Check sheet for the modelled part. Datum: model origin and axes. Units: mm. Give positions to 0.01 mm unless a question says otherwise; leave off trailing zeros. Write each loop counter-clockwise with the first axis right and the second up, starting at its lowest first coordinate (ties: lowest second). Pieces come first, ordered by that corner, then holes. Notation, with made-up numbers: (42, 89) -> (99, 89) arc R7 ccw to (99, 98) -> close; hole circle Ø3 at (75, 3.5). An arc over 180 degrees is marked (long way). Return JSON: item names as keys, results as strings.
from build123d import *

# Parameters (mm, degrees)
SKETCH1_W             = 225.5266
SKETCH1_H             = 171.6532
BOSS_EXTRUDE1_DEPTH   = 3.175
SKETCH2_W             = 19.05
SKETCH2_H             = 19.05
SKETCH2_W_2           = 28.702
CORNERCUT_DEPTH       = 4.175
SKETCH3_R             = 2.4257
MOUNTHOLES_DEPTH      = 4.175
F_8_CLEARANCE_HOLE1_D = 4.4958


with BuildPart() as part:
    # Sketch1 → Boss-Extrude1 (new body)
    with BuildSketch(Plane(origin=(0, 0, 0), x_dir=(1, 0, 0), z_dir=(0, 1, 0))):
        Rectangle(SKETCH1_W, SKETCH1_H)
    extrude(amount=BOSS_EXTRUDE1_DEPTH)

    # Sketch2 → CornerCut (cut, through all)
    with BuildSketch(Plane(origin=(0, 3.175, 0), x_dir=(1, 0, 0), z_dir=(0, 1, 0))):
        with Locations((-103.2383, 76.3016)):
            Rectangle(SKETCH2_W, SKETCH2_H)
        with Locations((98.4123, -76.3016)):
            Rectangle(SKETCH2_W_2, SKETCH2_H)
        with Locations((-103.2383, -76.3016)):
            Rectangle(SKETCH2_W, SKETCH2_H)
    extrude(amount=-CORNERCUT_DEPTH, mode=Mode.SUBTRACT)

    # Sketch3 → MountHoles (cut, through all)
    with BuildSketch(Plane(origin=(0, 3.175, 0), x_dir=(1, 0, 0), z_dir=(0, 1, 0))):
        with Locations((-103.2383, 57.6834)):
            Circle(SKETCH3_R)
        with Locations((-103.2383, -57.6834)):
            Circle(SKETCH3_R)
        with Locations((93.5863, -57.6834)):
            Circle(SKETCH3_R)
        with Locations((103.6701, 57.6834)):
            Circle(SKETCH3_R)
    extrude(amount=-MOUNTHOLES_DEPTH, mode=Mode.SUBTRACT)

    # #8 Clearance Hole1 (through all)
    with Locations(Plane(origin=(0, 3.175, 0), x_dir=(1, 0, 0), z_dir=(0, 1, 0))):
        with Locations((-44.629848387, -79.4766), (-24.2443, 17.982191502), (-71.4883, 17.982191502)):
            Hole(F_8_CLEARANCE_HOLE1_D / 2)


solid = part.part
(1) Cross-section at B-B on z = -70.5. Enter the section's corners in (x, y) (3 decimals), then the cut area to 3 significant figures.
Reply:
{"outline": "(-93.713, 0) -> (112.763, 0) -> (112.763, 3.175) -> (-93.713, 3.175) -> close", "area": "656 mm^2"}
(2) Thickness scan on L1, parallel to Z at x = -24.5, y = 3; L2, parallel to X at y = 1.8, z = -20 (3 decimals); L3, parallel to X at y = 1.45, z = -56. Record the ranges inside material, lowest first.
Reply:
{"L1": "-85.83 to -20.22, -15.75 to 85.83", "L2": "-112.763 to -72.479, -70.498 to -25.235, -23.254 to 112.763", "L3": "-112.76 to -104.98, -101.49 to 101.92, 105.42 to 112.76"}
(3) Depth check by flat-ended pin: pin 1 Ø3.5 at (x, z) = (-71.49, -17.98) entering from +Y; pin 2 Ø1 at (y, z) = (2, -80.5) entering from -X; pin 3 Ø5 at (x, z) = (-44.63, 79.48) entering from +Y (3 decimals); pin 4 Ø1.6 at (x, y) = (-101, 2) entering from -Z. Enter the tip coordinate at first touch or a pass-through.
Reply:
{"pin 1": "through", "pin 2": "x = -93.71", "pin 3": "y = 3.175", "pin 4": "z = -66.78"}
(4) Release check for a two-part mould opening along Z. For faces 1 (the cylindrical face through (104.97, 1.61, -59.73)), 2 (the flat face through (-2, 0, -1)), 3 (the cylindrical face through (-69.243, 1.565, -18.081)) record: pulls with the +Z half, pulls with the -Z half, needs draft (parallel to the pull), parting line crosses it, or undercut.
Reply:
{"face 1": "undercut", "face 2": "needs draft", "face 3": "undercut"}
(5) Cross-section at A-A on y = 1.2. Enter the section's corners in (x, z).
Reply:
{"outline": "(-112.76, -66.78) -> (-93.71, -66.78) -> (-93.71, -85.83) -> (112.76, -85.83) -> (112.76, 66.78) -> (84.06, 66.78) -> (84.06, 85.83) -> (-93.71, 85.83) -> (-93.71, 66.78) -> (-112.76, 66.78) -> close; hole circle Ø4.85 at (-103.24, -57.68); hole circle Ø4.85 at (-103.24, 57.68); hole circle Ø4.5 at (-71.49, -17.98); hole circle Ø4.5 at (-44.63, 79.48); hole circle Ø4.5 at (-24.24, -17.98); hole circle Ø4.85 at (93.59, 57.68); hole circle Ø4.85 at (103.67, -57.68)"}
